The model under review builds one solid part; all positions refer to its coordinate system, in mm. A direction names the side the tool comes from. Coordinates: 2 decimals unless noted, no trailing zeros. Order: outer loops, then holes, each group sorted by start corner. A loop starts at its lowest first (then second) coordinate and runs counter-clockwise, first axis right, second up. Notation, with made-up numbers: (86.5, 2) - (127.5, 2) arc R24 ccw to (127.5, 15) - close; hole circle Ø4 at (-33, 63). An arc over 180 degrees is marked (long way). Answer in a Markdown table with one row per item.
```python
from build123d import *

# Parameters (mm, degrees)
SKETCH1_W               = 70
SKETCH1_H               = 60
BOSS_EXTRUDE1_DEPTH     = 10
SKETCH2_W               = 60
SKETCH2_H               = 8
CUT_EXTRUDE1_DEPTH      = 55
SKETCH3_R               = 2.68983582
CUT_EXTRUDE2_DEPTH      = 55
MIRROR2_COPY_1_SKETCH_R = 2.68983582
MIRROR2_COPY_1_DEPTH    = 55


with BuildPart() as part:
    # Sketch1 → Boss-Extrude1 (new body)
    with BuildSketch(Plane(origin=(0, 0, 0), x_dir=(1, 0, 0), z_dir=(0, 1, 0))):
        with Locations((35, -30)):
            Rectangle(SKETCH1_W, SKETCH1_H)
    extrude(amount=BOSS_EXTRUDE1_DEPTH)

    # Sketch2 → Cut-Extrude1 (cut)
    with BuildSketch(Plane.XY.offset(60)):
        with Locations((35, 5)):
            Rectangle(SKETCH2_W, SKETCH2_H)
    extrude(amount=-CUT_EXTRUDE1_DEPTH, mode=Mode.SUBTRACT)

    # Sketch3 → Cut-Extrude2 (cut)
    with BuildSketch(Plane.ZY.offset(-65)):
        with Locations((10, 5)):
            Circle(SKETCH3_R)
    cut_extrude2 = extrude(amount=-CUT_EXTRUDE2_DEPTH, mode=Mode.SUBTRACT)

    # Mirror1: Cut-Extrude2 across plane
    add(cut_extrude2.mirror(Plane.ZY.offset(-35)), mode=Mode.SUBTRACT)

    # Mirror2: Cut-Extrude2 across plane
    add(cut_extrude2.mirror(Plane.XY.offset(30)), mode=Mode.SUBTRACT)

    # Mirror2 copy 1 sketch → Mirror2 copy 1 (cut)
    with BuildSketch(Plane(origin=(5, 0, 60), x_dir=(0, 0, -1), z_dir=(1, 0, 0))):
        with Locations((10, 5)):
            Circle(MIRROR2_COPY_1_SKETCH_R)
    extrude(amount=-MIRROR2_COPY_1_DEPTH, mode=Mode.SUBTRACT)


solid = part.part
```
Item 1: We need section B-B, the plane z = 36. Write out the cut boundary in (x, y), then the cut area to 3 significant figures.
Check values:
| item | result |
|---|---|
| outline | (0, 0) - (70, 0) - (70, 10) - (0, 10) - close; hole (5, 1) - (65, 1) - (65, 9) - (5, 9) - close |
| area | 220 mm^2 |
Item 2: To check wall thickness, follow line 1 (X direction, y = 7.75, z = 17.5); line 2 (Y direction, x = 41, z = 53); line 3 (Y direction, x = 3, z = 50). State the ranges of each line that lie inside material, in increasing order. Write a range as from..to.
Check values:
| item | result |
|---|---|
| line 1 | 0..5, 65..70 |
| line 2 | 0..1, 9..10 |
| line 3 | 0..2.31, 7.69..10 |
Item 3: We need section A-A, the plane z = 10. Write out the cut boundary in (x, y), then the cut area to 3 significant figures.
Check values:
| item | result |
|---|---|
| outline | (0, 0) - (70, 0) - (70, 2.31) - (65, 2.31) - (65, 1) - (5, 1) - (5, 2.31) - (0, 2.31) - close; (0, 7.69) - (5, 7.69) - (5, 9) - (65, 9) - (65, 7.69) - (70, 7.69) - (70, 10) - (0, 10) - close |
| area | 166 mm^2 |
Item 4: Tool access review of faces 4 (the face through (67.465, 3.97, 12.485)), 5 (the face through (65, 5, 33)): name each direction out of +Z, -Z, +X, -X, +Y, -Y from which nothing blocks a thin tool from reaching the whole face with its end or side.
Check values:
| item | result |
|---|---|
| face 4 | +X, -X |
| face 5 | +Z |
Item 5: We need section D-D, the plane x = 51.5. Write out the cut boundary in (y, z).
Check values:
| item | result |
|---|---|
| outline | (0, 0) - (10, 0) - (10, 60) - (9, 60) - (9, 5) - (1, 5) - (1, 60) - (0, 60) - close |
Item 6: We need section C-C, the plane y = 5. Write out the cut boundary in (x, z).
Check values:
| item | result |
|---|---|
| outline | (0, 0) - (70, 0) - (70, 7.31) - (65, 7.31) - (65, 5) - (5, 5) - (5, 7.31) - (0, 7.31) - close; (0, 12.69) - (5, 12.69) - (5, 47.31) - (0, 47.31) - close; (0, 52.69) - (5, 52.69) - (5, 60) - (0, 60) - close; (65, 12.69) - (70, 12.69) - (70, 47.31) - (65, 47.31) - close; (65, 52.69) - (70, 52.69) - (70, 60) - (65, 60) - close |
Item 7: Clearance check with a flat-ended pin moving along its axis: pin 1 Ø4.5 at (y, z) = (5, 50) entering from +X. State where the tip first meets the part, or that it passes through.
Check values:
| item | result |
|---|---|
| pin 1 | through |
Item 8: Mouldability with a two-part tool opening along X and no side actions: class faces 1 (the face through (0, 5, 30)), 2 (the face through (34.5, 9.4, 60)), 3 (the face through (35, 9, 33)) as +X half, -X half, draft (parallel to the pull), parting line (faces both ways), or undercut.
Check values:
| item | result |
|---|---|
| face 1 | -X half |
| face 2 | draft |
| face 3 | undercut |
